from build123d import *

# Parameters (mm, degrees)
SKETCH2_R          = 2.5
CUT_EXTRUDE1_DEPTH = 4
SKETCH3_R          = 3.075
CUT_EXTRUDE4_DEPTH = 87.539008545
SKETCH5_R          = 3.3
CUT_EXTRUDE6_DEPTH = 10
CHAMFER1_SIZE      = 1
SKETCH7_R          = 1
CUT_EXTRUDE8_DEPTH = 1


with BuildPart() as part:
    # Sketch1 → Revolve1 (revolve)
    with BuildSketch(Plane.XY, mode=Mode.PRIVATE) as revolve1_sk:
        Polygon((0, 60), (0, 33), (7, 33), (7, 26), (14, 26), (14, 23), (17, 23), (17, 60), align=None)
    revolve(revolve1_sk.sketch.rotate(Axis((0, 0, 0), (1, 0, 0)), 90), axis=Axis((0, 0, 0), (1, 0, 0)))

    # Sketch2 → Cut-Extrude1 (cut)
    with BuildSketch(Plane.ZY):
        with Locations((0, 40)):
            Circle(SKETCH2_R)
        with Locations((15.307337295, 36.9551813)):
            Circle(SKETCH2_R)
        with Locations((28.284271247, 28.284271247)):
            Circle(SKETCH2_R)
        with Locations((36.9551813, 15.307337295)):
            Circle(SKETCH2_R)
        with Locations((40, 0)):
            Circle(SKETCH2_R)
        with Locations((36.9551813, -15.307337295)):
            Circle(SKETCH2_R)
        with Locations((28.284271247, -28.284271247)):
            Circle(SKETCH2_R)
        with Locations((15.307337295, -36.9551813)):
            Circle(SKETCH2_R)
        with Locations((0, -40)):
            Circle(SKETCH2_R)
        with Locations((-15.307337295, -36.9551813)):
            Circle(SKETCH2_R)
        with Locations((-28.284271247, -28.284271247)):
            Circle(SKETCH2_R)
        with Locations((-36.9551813, -15.307337295)):
            Circle(SKETCH2_R)
        with Locations((-40, 0)):
            Circle(SKETCH2_R)
        with Locations((-36.9551813, 15.307337295)):
            Circle(SKETCH2_R)
        with Locations((-28.284271247, 28.284271247)):
            Circle(SKETCH2_R)
        with Locations((-15.307337295, 36.9551813)):
            Circle(SKETCH2_R)
    extrude(amount=-CUT_EXTRUDE1_DEPTH, mode=Mode.SUBTRACT)

    # Sketch3 → Cut-Extrude4 (cut, through all)
    with BuildSketch(Plane(origin=(17, 0, 0), x_dir=(0, 0, -1), z_dir=(1, 0, 0))):
        with Locations((49.03926402, -9.754516101)):
            Circle(SKETCH3_R)
        with Locations((16.071973265, -47.346506475)):
            Circle(SKETCH3_R)
        with Locations((-32.967290755, -37.591990374)):
            Circle(SKETCH3_R)
        with Locations((-49.03926402, 9.754516101)):
            Circle(SKETCH3_R)
        with Locations((-16.071973265, 47.346506475)):
            Circle(SKETCH3_R)
        with Locations((32.967290755, 37.591990374)):
            Circle(SKETCH3_R)
    extrude(amount=-CUT_EXTRUDE4_DEPTH, mode=Mode.SUBTRACT)

    # Sketch5 → Cut-Extrude6 (cut)
    with BuildSketch(Plane(origin=(17, 0, 0), x_dir=(0, 0, -1), z_dir=(1, 0, 0))):
        with Locations((32.967290755, 37.591990374)):
            Circle(SKETCH5_R)
        with Locations((49.03926402, -9.754516101)):
            Circle(SKETCH5_R)
        with Locations((16.071973265, -47.346506475)):
            Circle(SKETCH5_R)
        with Locations((-32.967290755, -37.591990374)):
            Circle(SKETCH5_R)
        with Locations((-49.03926402, 9.754516101)):
            Circle(SKETCH5_R)
        with Locations((-16.071973265, 47.346506475)):
            Circle(SKETCH5_R)
        with Locations((41.664925698, 14.143336473)):
            Circle(SKETCH5_R)
        with Locations((-8.583974169, -43.154552338)):
            Circle(SKETCH5_R)
        with Locations((-33.080951529, 29.011215864)):
            Circle(SKETCH5_R)
    extrude(amount=-CUT_EXTRUDE6_DEPTH, mode=Mode.SUBTRACT)

    # Chamfer1
    chamfer1_edges = [part.edges().sort_by_distance(p)[0] for p in [
        (17, -9.754516101, -45.73926402),
        (17, -47.346506475, -12.771973265),
        (17, -37.591990374, 36.267290755),
        (17, 9.754516101, 52.33926402),
        (17, 29.011215864, 36.380951529),
        (17, -43.154552338, 11.883974169),
        (17, 14.143336473, -38.364925698),
        (17, 47.346506475, 19.371973265),
        (17, 37.591990374, -29.667290755),
    ]]
    chamfer(chamfer1_edges, length=CHAMFER1_SIZE)

    # Sketch7 → Cut-Extrude8 (cut)
    with BuildSketch(Plane.ZY):
        with Locations((39.086428505, -31.895390573)):
            Circle(SKETCH7_R)
    extrude(amount=-CUT_EXTRUDE8_DEPTH, mode=Mode.SUBTRACT)


solid = part.part
Verification items for the finished model (mm, model axes). A direction names the side the tool comes from. Give positions to 0.01 mm unless a question says otherwise; leave off trailing zeros. Order: outer loops, then holes, each group sorted by start corner. A loop starts at its lowest first (then second) coordinate and runs counter-clockwise, first axis right, second up. Notation, with made-up numbers: M -1.5,63.25 L 6.5,63.25 A20 ccw 6.5,82.25 Z; hole C 83.5,25.5 d11. An arc over 180 degrees is marked long. Use one line per item in the form item = value. Start each with the question number.
Q1. Mould release check, pull along Y, two halves, no side actions. Record for faces 1 (the flat face through (0, 26, 26)), 2 (the cylindrical face through (1.972, -39.396, -15.849)): +Y half, -Y half, draft (parallel to the pull), parting line (faces both ways), or undercut.
Q2. Go/stop test with flat-tipped pins: pin 1 Ø7.5 at (y, z) = (29.01, 33.08) entering from +X; pin 2 Ø8 at (y, z) = (-37.59, 32.97) entering from +X; pin 3 Ø1.5 at (x, y) = (4, -19) entering from -Z; pin 4 Ø5.5 at (y, z) = (-47.35, -16.07) entering from +X. Record where each tip stops, or that it passes through.
Q3. Access from +Z, -Z, +X, -X, +Y, -Y to the whole of each face (thin tool, end or side, straight path). Record for faces 3 (the flat face through (14, 21, 10)), 4 (the cylindrical face through (11.563, 44.125, 16.787)), 5 (the cylindrical face through (3.549, 47.482, 19.144)).
Q4. Section check A-A (y = 0). Enter the section's corners in (x, z).
Q5. Scan lines: line 1 along Y through (x, z) = (3.05, 0); line 2 along Z through (x, y) = (1.75, 35.5); line 3 along Z through (x, y) = (5.75, 12.5). Record each from-to range of solid material in increasing order. Write a range as [from, to].
Q6. Section check B-B (x = 11.75). Count the separate pieces of the cut face and the enclosed holes in it, then the cut area to 3 significant figures.
Evaluation:
q1.face_1 = draft
q1.face_2 = undercut
q2.pin_1 = 16.45
q2.pin_2 = 16.7
q2.pin_3 = -57.16
q2.pin_4 = through
q3.face_3 = -X
q3.face_4 = +X
q3.face_5 = +X, -X
q4.outline = M 0,-60 L 17,-60 L 17,-23 L 14,-23 L 14,-26 L 7,-26 L 7,-33 L 0,-33 L 0,-37.5 L 4,-37.5 L 4,-42.5 L 0,-42.5 Z; M 0,33 L 7,33 L 7,26 L 14,26 L 14,23 L 17,23 L 17,60 L 0,60 L 0,42.5 L 4,42.5 L 4,37.5 L 0,37.5 Z
q5.line_1 = [-60, -42.5], [-37.5, -33], [33, 37.5], [42.5, 60]
q5.line_2 = [-48.37, -35.22], [-30.71, -17.34], [-13.27, 13.27], [17.34, 48.37]
q5.line_3 = [-58.68, -30.54], [30.54, 47.65], [50.42, 58.68]
q6.separate_pieces = 1
q6.enclosed_holes = 10
q6.area = 8,880 mm2
